Geometry check sheet. Reference: the model listing, model coordinates, mm. Coordinates: 2 decimals unless noted, no trailing zeros. Loops run counter-clockwise (first coordinate to the right, second up) from the corner with the lowest first, then second, coordinate; pieces in that order, holes last.
from build123d import *

# Parameters (mm, degrees)
SKETCH1_W                      = 110.56
SKETCH1_H                      = 42
BOSS_EXTRUDE1_DEPTH            = 2
F_2_2_2_2_DIAMETER_HOLE1_D     = 2.2
F_2_2_2_2_DIAMETER_HOLE1_DEPTH = 2


with BuildPart() as part:
    # Sketch1 → Boss-Extrude1 (new body)
    with BuildSketch(Plane(origin=(0, 0, 0), x_dir=(1, 0, 0), z_dir=(0, 1, 0))):
        Rectangle(SKETCH1_W, SKETCH1_H)
    extrude(amount=BOSS_EXTRUDE1_DEPTH)

    # Ø2.2 (2.2) Diameter Hole1
    with Locations(Plane(origin=(0, 0, 0), x_dir=(-1, 0, 0), z_dir=(0, -1, 0))):
        with Locations((53.28, -19.5), (53.28, 19.5), (-52.78, 19.5), (-0.579521869, 19.5), (-0.579521869, -19.5), (-52.78, -19.5)):
            Hole(F_2_2_2_2_DIAMETER_HOLE1_D / 2, depth=F_2_2_2_2_DIAMETER_HOLE1_DEPTH)


solid = part.part
1) Section check A-A on z = 19.5. Record the cut outline in (x, y), and give its area (3 significant figures).
Data:
outline: (-55.28, 0) - (-54.38, 0) - (-54.38, 2) - (-55.28, 2) - close; (-52.18, 0) - (-0.52, 0) - (-0.52, 2) - (-52.18, 2) - close; (1.68, 0) - (51.68, 0) - (51.68, 2) - (1.68, 2) - close; (53.88, 0) - (55.28, 0) - (55.28, 2) - (53.88, 2) - close
area: 208 mm2
2) Depth check by flat-ended pin: pin 1 (1.3 mm diameter, centred on x = -53.28, z = -19.5, fed in from +Y). Enter the tip coordinate at first touch or a pass-through.
Data:
pin 1: passes through
3) Material ranges on probe 1 along X at (y, z) = (0.9, -19.5); probe 2 along Z at (x, y) = (-53.28, 0.6), recorded low to high.
Data:
probe 1: x = -55.28 to -54.38, -52.18 to -0.52, 1.68 to 51.68, 53.88 to 55.28
probe 2: z = -21 to -20.6, -18.4 to 18.4, 20.6 to 21
4) Section check B-B on x = 52.78. Record the cut outline in (y, z).
Data:
outline: (0, -21) - (2, -21) - (2, -20.6) - (0, -20.6) - close; (0, -18.4) - (2, -18.4) - (2, 18.4) - (0, 18.4) - close; (0, 20.6) - (2, 20.6) - (2, 21) - (0, 21) - close
5) Mould release check, pull along Z, two halves, no side actions. Record for faces 1 (the cylindrical face through (0.341, 1.014, 20.574)), 2 (the flat face through (-1, 1, 21)), 3 (the flat face through (-55.28, 1, 0)): +Z half, -Z half, draft (parallel to the pull), parting line (faces both ways), or undercut.
Data:
face 1: undercut
face 2: +Z half
face 3: draft
